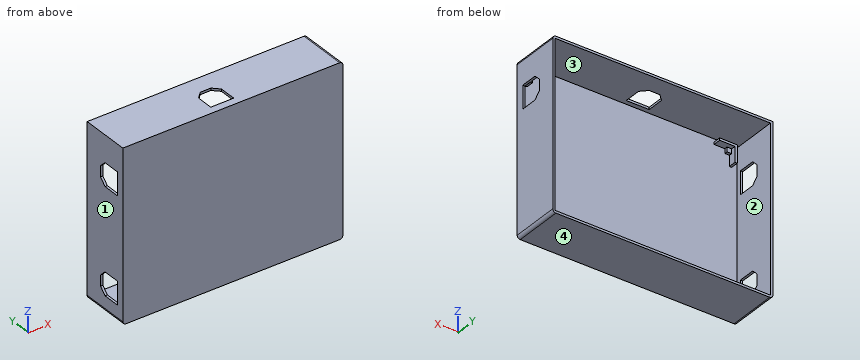
```python
from build123d import *

# Parameters (mm, degrees)
SKETCH1_W                = 1600
SKETCH1_H                = 1600
BOSS_EXTRUDE1_DEPTH      = 2
SKETCH2_R                = 1.585
BOSS_EXTRUDE2_DEPTH      = 5
SKETCH3_W                = 1.5
SKETCH3_H                = 10.8
SKETCH3_H_2              = 16.825
BOSS_EXTRUDE3_DEPTH      = 30
CUT_EXTRUDE1_DEPTH       = 1132.768527571
CUT_EXTRUDE1_DEPTH_BACK  = 1132.768527571
SKETCH5_OUTSIDE_W        = 2054.594
SKETCH5_OUTSIDE_H        = 2054.594
SKETCH5_OUTSIDE_W_2      = 200
SKETCH5_OUTSIDE_H_2      = 200
SKETCH6_W                = 200
SKETCH6_H                = 97
BOSS_EXTRUDE4_DEPTH      = 2
BOSS_EXTRUDE6_DEPTH      = 30
CUT_EXTRUDE7_START       = -2
CUT_EXTRUDE7_DEPTH       = 32
SKETCH15_W               = 48.54
SKETCH15_H               = 10.95
BOSS_EXTRUDE8_DEPTH      = 1.5
CHAMFER1_SIZE            = 3
CUT_EXTRUDE9_DEPTH       = 1132.768527571
CUT_EXTRUDE9_DEPTH_BACK  = 1132.768527571
SKETCH16_W               = 83.170959918
SKETCH16_H               = 74.318470717
BOSS_EXTRUDE9_DEPTH      = 30
CUT_EXTRUDE8_DEPTH       = 814.397965328
CUT_EXTRUDE8_DEPTH_BACK  = 814.397965328
SKETCH18_W               = 20.53541424
SKETCH18_H               = 18.617271152
BOSS_EXTRUDE10_DEPTH     = 1.5
BOSS_EXTRUDE11_DEPTH     = 5
SKETCH20_W               = 3
SKETCH20_H               = 3
BOSS_EXTRUDE12_DEPTH     = 2
FILLET1_R                = 2
BOSS_EXTRUDE13_DEPTH     = 30
CUT_EXTRUDE10_DEPTH      = 1132.823307765
CUT_EXTRUDE10_DEPTH_BACK = 1132.823307765
SKETCH22_W               = 118.842145749
SKETCH22_H               = 72.51699158
CUT_EXTRUDE11_DEPTH      = 20


# Read off the part's stored shape, not the designer's step: Cut-Extrude7
with BuildPart() as part:
    # Sketch1 → Boss-Extrude1 (new body)
    with BuildSketch(Plane(origin=(0, 0, 0), x_dir=(1, 0, 0), z_dir=(0, 1, 0))):
        Rectangle(SKETCH1_W, SKETCH1_H)
    extrude(amount=BOSS_EXTRUDE1_DEPTH)

    # Sketch2 → Boss-Extrude2 (add)
    with BuildSketch(Plane(origin=(0, 2, 0), x_dir=(1, 0, 0), z_dir=(0, 1, 0))):
        with Locations(Location((-782.85, -746.2, 0), (0, 0, 270))):
            Circle(SKETCH2_R)
        with Locations(Location((-732.05, -761.44, 0), (0, 0, 270))):
            Circle(SKETCH2_R)
        with Locations(Location((-784.12, -794.46, 0), (0, 0, 270))):
            Circle(SKETCH2_R)
        with Locations(Location((-732.05, -789.38, 0), (0, 0, 270))):
            Circle(SKETCH2_R)
    extrude(amount=BOSS_EXTRUDE2_DEPTH)

    # Sketch3 → Boss-Extrude3 (add)
    with BuildSketch(Plane(origin=(0, 2, 0), x_dir=(1, 0, 0), z_dir=(0, 1, 0))):
        with Locations((-799.25, -746.06)):
            Rectangle(SKETCH3_W, SKETCH3_H)
        Polygon((-798.5, -800), (-800, -800), (-800, -795.325), (-798.5, -795.325), (-798.5, -798.5), (-648.5, -798.5), (-648.5, -800), align=None)
        with Locations((-799.25, -774.9125)):
            Rectangle(SKETCH3_W, SKETCH3_H_2)
    extrude(amount=BOSS_EXTRUDE3_DEPTH)

    # Sketch5 outside → Cut-Extrude1 (cut, two sides: drawn at the far end of the back side and taken through both)
    with BuildSketch(Plane(origin=(0, 2, 0), x_dir=(1, 0, 0), z_dir=(0, 1, 0)).offset(-CUT_EXTRUDE1_DEPTH_BACK)):
        Rectangle(SKETCH5_OUTSIDE_W, SKETCH5_OUTSIDE_H)
        with Locations((-700, -700)):
            Rectangle(SKETCH5_OUTSIDE_W_2, SKETCH5_OUTSIDE_H_2, mode=Mode.SUBTRACT)
    extrude(amount=CUT_EXTRUDE1_DEPTH + CUT_EXTRUDE1_DEPTH_BACK, mode=Mode.SUBTRACT)

    # Sketch6 → Boss-Extrude4 (add)
    with BuildSketch(Plane(origin=(0, 2, 0), x_dir=(1, 0, 0), z_dir=(0, 1, 0))):
        with Locations((-698.5, -652.5)):
            Rectangle(SKETCH6_W, SKETCH6_H)
    extrude(amount=-BOSS_EXTRUDE4_DEPTH)

    # Sketch7 → Boss-Extrude6 (add)
    with BuildSketch(Plane(origin=(0, 2, 0), x_dir=(1, 0, 0), z_dir=(0, 1, 0))):
        Polygon((-798.5, -740.66), (-798.5, -601.5), (-601.5, -601.5), (-601.5, -605.5), (-600, -605.5), (-600, -699.5), (-601.5, -699.5), (-601.5, -798.5), (-648.5, -798.5), (-648.5, -800), (-600, -800), (-600, -701), (-598.5, -701), (-598.5, -604), (-600, -604), (-600, -600), (-800, -600), (-800, -740.66), align=None)
    extrude(amount=BOSS_EXTRUDE6_DEPTH)

    # Cut-Extrude7 outline → Cut-Extrude7 (cut)
    with BuildSketch(Plane(origin=(0, 2, 0), x_dir=(1, 0, 0), z_dir=(0, 1, 0)).offset(CUT_EXTRUDE7_START)):
        Polygon((-656.5, -632.91), (-656.5, -800), (-600, -800), (-600, -701), (-598.5, -701), (-598.5, -604), (-600, -604), (-600, -600), (-800, -600), (-800, -632.91), align=None)
    extrude(amount=CUT_EXTRUDE7_DEPTH, mode=Mode.SUBTRACT)

    # Sketch15 → Boss-Extrude8 (add)
    with BuildSketch(Plane.ZY.offset(800)):
        with Locations((775.73, 26.525)):
            Rectangle(SKETCH15_W, SKETCH15_H)
    extrude(amount=-BOSS_EXTRUDE8_DEPTH)

    # Chamfer1
    chamfer1_edges = [part.edges().sort_by_distance(p)[0] for p in [
        (-799.25, 21.05, 766.5),
        (-799.25, 21.05, 795.325),
        (-799.25, 21.05, 751.46),
        (-799.25, 21.05, 783.325),
    ]]
    chamfer(chamfer1_edges, length=CHAMFER1_SIZE)

    # Sketch16 → Cut-Extrude9 (cut, two sides: drawn at the far end of the back side and taken through both)
    with BuildSketch(Plane(origin=(0, 2, 0), x_dir=(1, 0, 0), z_dir=(0, 1, 0)).offset(-CUT_EXTRUDE9_DEPTH_BACK)):
        with Locations((-682.924520041, -781.069235359)):
            Rectangle(SKETCH16_W, SKETCH16_H)
    extrude(amount=CUT_EXTRUDE9_DEPTH + CUT_EXTRUDE9_DEPTH_BACK, mode=Mode.SUBTRACT)

    # Sketch17 → Boss-Extrude9 (add)
    with BuildSketch(Plane(origin=(0, 2, 0), x_dir=(1, 0, 0), z_dir=(0, 1, 0))):
        Polygon((-798.5, -632.91), (-656.5, -632.91), (-656.5, -743.91), (-724.51, -743.91), (-724.51, -800), (-726.01, -800), (-726.01, -742.41), (-658, -742.41), (-658, -634.41), (-798.5, -634.41), align=None)
    extrude(amount=BOSS_EXTRUDE9_DEPTH)

    # Sketch14 → Cut-Extrude8 (cut, two sides: drawn at the far end of the back side and taken through both)
    with BuildSketch(Plane.ZY.offset(800).offset(-CUT_EXTRUDE8_DEPTH_BACK)):
        Polygon((642.91, 5), (657.91, 5), (657.91, 16), (653.91, 20), (646.91, 20), (642.91, 16), align=None)
        Polygon((711.46, 5), (726.46, 5), (726.46, 16), (722.46, 20), (715.46, 20), (711.46, 16), align=None)
    extrude(amount=CUT_EXTRUDE8_DEPTH + CUT_EXTRUDE8_DEPTH_BACK, mode=Mode.SUBTRACT)

    # Sketch18 → Boss-Extrude10 (add)
    with BuildSketch(Plane(origin=(-656.5, 0, 0), x_dir=(0, 0, -1), z_dir=(1, 0, 0))):
        with Locations((-651.07097558, 11.926550953)):
            Rectangle(SKETCH18_W, SKETCH18_H)
    extrude(amount=-BOSS_EXTRUDE10_DEPTH)

    # Sketch19 → Boss-Extrude11 (add)
    with BuildSketch(Plane(origin=(0, 2, 0), x_dir=(1, 0, 0), z_dir=(0, 1, 0))):
        Polygon((-793.5, -647.91), (-795, -647.91), (-795, -636.41), (-783.5, -636.41), (-783.5, -637.91), (-793.5, -637.91), align=None)
        Polygon((-661.5, -647.91), (-660, -647.91), (-660, -636.41), (-671.5, -636.41), (-671.5, -637.91), (-661.5, -637.91), align=None)
        Polygon((-661.5, -728.91), (-658, -728.91), (-658, -742.41), (-671.5, -742.41), (-671.5, -738.91), (-661.5, -738.91), align=None)
        Polygon((-793.5, -728.91), (-795, -728.91), (-795, -740.41), (-783.5, -740.41), (-783.5, -738.91), (-793.5, -738.91), align=None)
    extrude(amount=BOSS_EXTRUDE11_DEPTH)

    # Sketch20 → Boss-Extrude12 (add)
    with BuildSketch(Plane(origin=(0, 2, 0), x_dir=(1, 0, 0), z_dir=(0, 1, 0))):
        with Locations((-792, -639.41)):
            Rectangle(SKETCH20_W, SKETCH20_H)
        with Locations((-663, -639.41)):
            Rectangle(SKETCH20_W, SKETCH20_H)
        with Locations((-663, -737.41)):
            Rectangle(SKETCH20_W, SKETCH20_H)
        with Locations((-792, -737.41)):
            Rectangle(SKETCH20_W, SKETCH20_H)
    extrude(amount=BOSS_EXTRUDE12_DEPTH)

    # Fillet1
    fillet1_edges = [part.edges().sort_by_distance(p)[0] for p in [
        (-656.5, 16, 632.91),
        (-800, 16, 632.91),
        (-656.5, 16, 743.91),
        (-724.51, 16, 800),
        (-724.51, 16, 743.91),
        (-800, 16, 800),
    ]]
    fillet(fillet1_edges, radius=FILLET1_R)

    # Sketch21 → Boss-Extrude13 (add)
    with BuildSketch(Plane(origin=(0, 2, 0), x_dir=(1, 0, 0), z_dir=(0, 1, 0))):
        Polygon((-726.01, -742.41), (-798.5, -742.41), (-800, -743.91), (-720.182968703, -743.91), align=None)
    extrude(amount=BOSS_EXTRUDE13_DEPTH)

    # Sketch22 → Cut-Extrude10 (cut, two sides: drawn at the far end of the back side and taken through both)
    with BuildSketch(Plane(origin=(0, 32, 0), x_dir=(1, 0, 0), z_dir=(0, 1, 0)).offset(-CUT_EXTRUDE10_DEPTH_BACK)):
        with Locations((-761.569685202, -780.16849579)):
            Rectangle(SKETCH22_W, SKETCH22_H)
    extrude(amount=CUT_EXTRUDE10_DEPTH + CUT_EXTRUDE10_DEPTH_BACK, mode=Mode.SUBTRACT)

    # Sketch23 → Cut-Extrude11 (cut)
    with BuildSketch(Plane.XY.offset(743.91)):
        Polygon((-735, 20), (-728, 20), (-724, 16), (-724, 5), (-739, 5), (-739, 16), align=None)
    extrude(amount=-CUT_EXTRUDE11_DEPTH, mode=Mode.SUBTRACT)


solid = part.part
```
Input: part model. Units: mm. Frame: model coordinates. Face numbers are marked on the shaded views. Coordinates: 2 decimals unless noted, no trailing zeros. Order: outer loops, then holes, each group sorted by start corner. A loop starts at its lowest first (then second) coordinate and runs counter-clockwise, first axis right, second up. Notation, with made-up numbers: (47, 69.25) - (71, 69.25) arc R32 ccw to (71, 100.25) - close; hole circle Ø2 at (-21.75, 61.5). An arc over 180 degrees is marked (long way). Return JSON: item names as keys, results as strings.
Q1. Cut plane B-B (y = 25). Return loops of the section in (x, z), then the cut area to 3 significant figures.
The answers:
{"outline": "(-800, 634.91) arc R2 ccw to (-798, 632.91) - (-658.5, 632.91) arc R2 ccw to (-656.5, 634.91) - (-656.5, 741.91) arc R2 ccw to (-658.5, 743.91) - (-800, 743.91) - close; hole (-798.5, 634.41) - (-658, 634.41) - (-658, 742.41) - (-798.5, 742.41) - close", "area": "752 mm2"}
Q2. Cut plane C-C (z = 704.5). Return loops of the section in (x, y), then the cut area to 3 significant figures.
The answers:
{"outline": "(-800, 0) - (-656.5, 0) - (-656.5, 32) - (-658, 32) - (-658, 2) - (-798.5, 2) - (-798.5, 32) - (-800, 32) - close", "area": "377 mm2"}
Q3. Draft query along X for the marked faces 1, 2, 3 and 4. Return one class per face: +X half, -X half, draft (parallel to the pull), parting line (faces both ways), or undercut.
The answers:
{"face 1": "-X half", "face 2": "undercut", "face 3": "undercut", "face 4": "draft"}
Q4. Ray query, probe 1 along X at (y, z) = (14, 689); probe 2 along Z at (x, y) = (-731, 3.5); probe 3 along X at (y, z) = (6, 641). Return the intervals inside material, ascending.
The answers:
{"probe 1": "x = -800 to -798.5, -658 to -656.5", "probe 2": "z = 632.91 to 634.41, 742.41 to 743.91", "probe 3": "x = -800 to -798.5, -795 to -793.5, -661.5 to -660, -658 to -656.5"}
Q5. Cut plane D-D (x = -788). Return loops of the section in (y, z), then the cut area to 3 significant figures.
The answers:
{"outline": "(0, 632.91) - (32, 632.91) - (32, 634.41) - (2, 634.41) - (2, 636.41) - (7, 636.41) - (7, 637.91) - (2, 637.91) - (2, 738.91) - (7, 738.91) - (7, 740.41) - (2, 740.41) - (2, 742.41) - (32, 742.41) - (32, 743.91) - (0, 743.91) - close", "area": "327 mm2"}
Q6. Cut plane A-A (y = 17.5). Return loops of the section in (x, z).
The answers:
{"outline": "(-800, 634.91) arc R2 ccw to (-798, 632.91) - (-658.5, 632.91) arc R2 ccw to (-656.5, 634.91) - (-656.5, 712.96) - (-658, 712.96) - (-658, 634.41) - (-798.5, 634.41) - (-798.5, 644.41) - (-800, 644.41) - close; (-800, 656.41) - (-798.5, 656.41) - (-798.5, 712.96) - (-800, 712.96) - close; (-800, 724.96) - (-798.5, 724.96) - (-798.5, 742.41) - (-737.5, 742.41) - (-737.5, 743.91) - (-800, 743.91) - close; (-725.5, 742.41) - (-658, 742.41) - (-658, 724.96) - (-656.5, 724.96) - (-656.5, 741.91) arc R2 ccw to (-658.5, 743.91) - (-725.5, 743.91) - close"}
Q7. First-contact query: pin 1 (2 mm diameter, centred on y = 15, z = 725, fed in from +X); pin 2 (0.9 mm diameter, centred on x = -662.5, z = 640, fed in from +Y); pin 3 (6 mm diameter, centred on x = -788.5, z = 736.5, fed in from +Y); pin 4 (4 mm diameter, centred on x = -724.5, z = 731.5, fed in from +Y). Flat tips, straight axial feed; report the tip coordinate or a pass-through.
The answers:
{"pin 1": "passes through", "pin 2": "stops at y = 4", "pin 3": "stops at y = 7", "pin 4": "stops at y = 2"}
